from build123d import *

# Parameters (mm, degrees)
F0_W           = 171
F0_H           = 206.193
F1_DEPTH       = 18
F2_D           = 32
F4_DEPTH       = 171.001
F6_D           = 4
F6_CSINK_D     = 8.2
F6_CSINK_ANGLE = 90
F7_D           = 4
F7_CSINK_D     = 8.2
F7_CSINK_ANGLE = 90
F8_D           = 4
F8_CSINK_D     = 8.2
F8_CSINK_ANGLE = 90
F9_D           = 4
F9_CSINK_D     = 8.2
F9_CSINK_ANGLE = 90


with BuildPart() as f1:
    # F0 (on Front) → F1 (new body)
    with BuildSketch(Plane.XZ):
        Rectangle(F0_W, F0_H)
    extrude(amount=F1_DEPTH)

    # F2 (through all)
    with Locations(Plane(origin=(0, 0, 0), x_dir=(1, 0, 0), z_dir=(0, 1, 0))):
        with Locations((0, -66.9035)):
            Hole(F2_D / 2)

    # F3 (on face) → F4 (cut, through all)
    with BuildSketch(Plane(origin=(-85.5, 0, 0), x_dir=(0, -1, 0), z_dir=(-1, 0, 0))):
        Polygon((18, 103.0965), (0, 103.0965), (18, 99.9226143472), align=None)
    extrude(amount=-F4_DEPTH, mode=Mode.SUBTRACT)

    # F6 (through all)
    with Locations(Plane.XZ.offset(18)):
        with Locations((0, -76.0965)):
            CounterSinkHole(F6_D / 2, F6_CSINK_D / 2, counter_sink_angle=F6_CSINK_ANGLE)

    # F7 (through all)
    with Locations(Plane.XZ.offset(18)):
        with Locations((-76.5, -76.0965), (76.5, -76.0965)):
            CounterSinkHole(F7_D / 2, F7_CSINK_D / 2, counter_sink_angle=F7_CSINK_ANGLE)

    # F8 (through all)
    with Locations(Plane.XZ.offset(18)):
        with Locations((-76.5, 81.9035), (76.5, 81.9035)):
            CounterSinkHole(F8_D / 2, F8_CSINK_D / 2, counter_sink_angle=F8_CSINK_ANGLE)

    # F9 (through all)
    with Locations(Plane.XZ.offset(18)):
        with Locations((-76.5, 2.9035), (76.5, 2.9035)):
            CounterSinkHole(F9_D / 2, F9_CSINK_D / 2, counter_sink_angle=F9_CSINK_ANGLE)


solid = f1.part
Part model, mm, in its own coordinate system. Give positions to 0.01 mm unless a question says otherwise; leave off trailing zeros. Order: outer loops, then holes, each group sorted by start corner. A loop starts at its lowest first (then second) coordinate and runs counter-clockwise, first axis right, second up. Notation, with made-up numbers: (-13.5, -32.75) - (22.5, -32.75) arc R34 ccw to (22.5, 0.25) - close; hole circle Ø2 at (78.5, 71.25). An arc over 180 degrees is marked (long way). One line per question, with ' | ' between items.
1. Drill centre lines: probe 1 along Z at (x, y) = (0, -5.75); probe 2 along X at (y, z) = (-7.5, -75); probe 3 along X at (y, z) = (-6.25, 83). Where is each one in solid material? Low to high.
Filled in:
probe 1: -103.1 to -78.1, -74.1 to 50.9, 82.9 to 102.08 | probe 2: -85.5 to -78.17, -74.83 to -1.67, 1.67 to 74.83, 78.17 to 85.5 | probe 3: -85.5 to -78.17, -74.83 to 74.83, 78.17 to 85.5
2. Band-saw the part on B-B on y = -7.5. Give the number of separate pieces and of enclosed holes in the cut face, then the cut area to 3 significant figures.
Filled in:
separate pieces: 1 | enclosed holes: 8 | area: 34,100 mm²
3. Band-saw the part on A-A on z = 63.5. List the corners of the cut face in (x, y), then the cut area to 3 significant figures.
Filled in:
outline: (-85.5, -18) - (-15.63, -18) - (-15.63, 0) - (-85.5, 0) - close; (15.63, -18) - (85.5, -18) - (85.5, 0) - (15.63, 0) - close | area: 2,520 mm²
4. Drop flat-ended pins along their axis: P1, Ø2, axis at x = 29, y = -13, coming from the +Z side; P2, Ø5, axis at x = 0, z = -76.1, coming from the -Y side; P3, Ø4, axis at x = 3, y = -11.5, coming from the +Z side. Give the stop position or say it passes through.
Filled in:
P1: z = 100.98 | P2: y = -16.4 | P3: z = 101.42
5. Pull direction X, two halves, no side cores. Call faces 1 (the face through (85.5, -9, -1)), 2 (the face through (-1, -18, 0)), 3 (the face through (-7.38, -9.13, 81.1)): +X half, -X half, draft (parallel to the pull), parting line (faces both ways), or undercut.
Filled in:
face 1: +X half | face 2: draft | face 3: undercut
